For this review, use the dimensioned drawing (mm, ordinates from the lowest corner) and the shaded views. Give positions to 0.01 mm unless a question says otherwise; leave off trailing zeros. Write each loop counter-clockwise with the first axis right and the second up, starting at its lowest first coordinate (ties: lowest second). Pieces come first, ordered by that corner, then holes. Notation, with made-up numbers: (0.5, -26.75) - (16.5, -26.75) arc R18 cw to (16.5, -18.75) - close; hole circle Ø2 at (-35.5, -3.75). An arc over 180 degrees is marked (long way). Use a Markdown table: item, result. Add a question column.
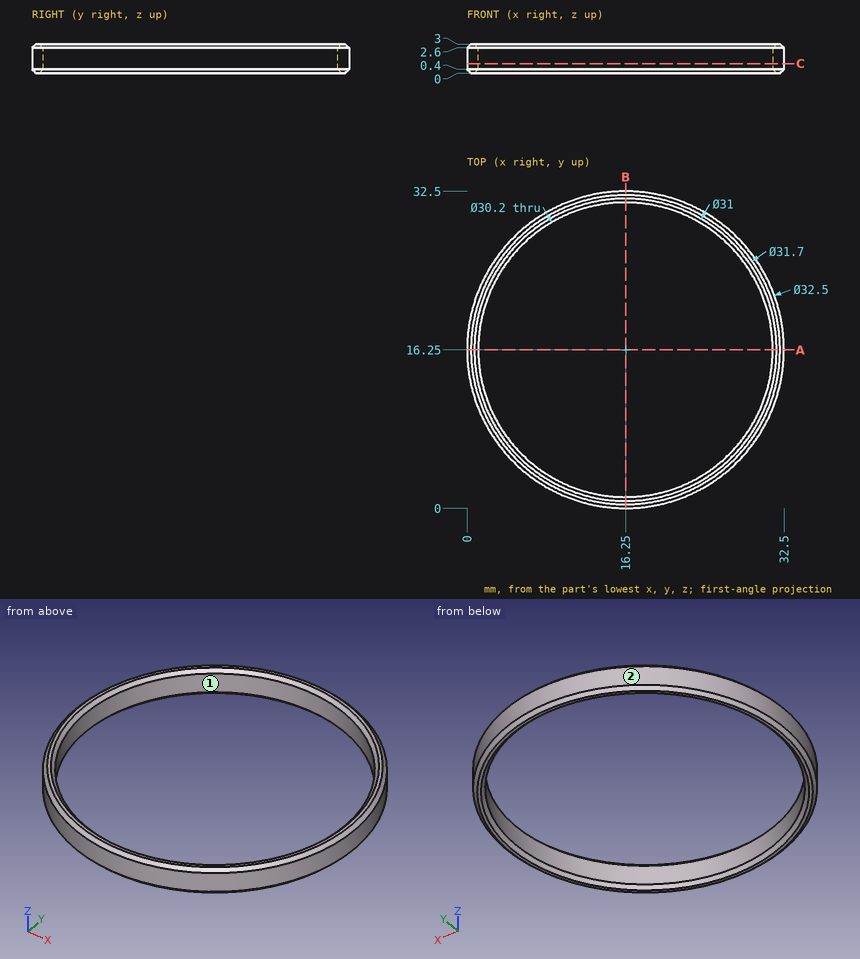
(1) Add section A-A (y = 16.25). State the section outline as (x, z) points.
(2) Mouldability with a two-part tool opening along X and no side actions: class the marked faces 1 and 2 as +X half, -X half, draft (parallel to the pull), parting line (faces both ways), or undercut.
(3) For line 1 along Y through (x, z) = (16.25, 1.4); line 2 along X through (y, z) = (5, 1.35); line 3 along Y through (x, z) = (7, 2), list the stretches that pass through material, from the lowest coordinate up.
(4) Add section C-C (z = 1). State the section outline as (x, y) points.
(5) Insertion check: pin 1 (1 mm diameter, centred on y = 17, z = 2.5, fed in from +X). The pin has a flat end and moves straight along its axis. Give the tip position at first contact, or say it passes through.
Answers follow:
| question | item | result |
|---|---|---|
| 1 | outline | (0, 0.4) - (0.4, 0) - (0.75, 0) - (1.15, 0.4) - (1.15, 2.6) - (0.75, 3) - (0.4, 3) - (0, 2.6) - close; (31.35, 0.4) - (31.75, 0) - (32.1, 0) - (32.5, 0.4) - (32.5, 2.6) - (32.1, 3) - (31.75, 3) - (31.35, 2.6) - close |
| 2 | face 1 | undercut |
| 2 | face 2 | parting line |
| 3 | line 1 | 0 to 1.15, 31.35 to 32.5 |
| 3 | line 2 | 4.52 to 6.18, 26.32 to 27.98 |
| 3 | line 3 | 2.89 to 4.31, 28.19 to 29.61 |
| 4 | outline | circle Ø32.5 at (16.25, 16.25); hole circle Ø30.2 at (16.25, 16.25) |
| 5 | pin 1 | x = 32.5 |
